Autodesk Inventor part; units mm, degrees
ref_plane "YZ Plane" through (0, 0, 0) normal (1, 0, 0) x (0, 1, 0)
ref_plane "XZ Plane" through (0, 0, 0) normal (0, 1, 0) x (-1, 0, 0)
ref_plane "XY Plane" through (0, 0, 0) normal (0, 0, 1) x (1, 0, 0)
sketch "Sketch1" plane through (0, 0, 0) normal (0, 0, 1) x (1, 0, 0)
  line L0 (-17.0246, -1.3061) -> (-17.0246, -8.9261)
  line L1 (-17.0246, -8.9261) -> (-15.272, -8.9261)
  line L2 (-15.272, -8.9261) -> (-15.272, -2.5761)
  line L3 (-15.272, -2.5761) -> (-13.8496, -2.5761)
  line L4 (-13.8496, -2.5761) -> (-13.8496, -1.9411)
  arc A0 (-13.8496, -1.9411) -> (-17.0246, -1.3061) centre (-17.0246, -9.5611) ccw
  dimension "length" = 6.35
  dimension "d1" = 0.635
  dimension "d2" = 1.27
  dimension "d3" = 1.7526
  dimension "d4" = 3.175
revolve "Revolution1" add sketch "Sketch1" angle 360 about axis through (-17.0246, -1.3061, 0) along (0, -1, 0)
ref_plane "Work Plane1" through (-17.0246, -1.3061, 0) normal (0, -1, 0) x (1, 0, 0)
sketch "Sketch2" plane through (-17.0246, -1.3061, 0) normal (0, -1, 0) x (1, 0, 0)
  line L0 (-3.0822, -0.762) -> (3.0822, -0.762)
  circle A0 centre (0, 0) radius 0.762 construction
  circle A1 centre (0, 0) radius 3.175
  line L1 (-3.0822, 0.762) -> (3.0822, 0.762)
  dimension "d8" = 1.524
extrude "Extrusion1" cut sketch "Sketch2" along normal blind 0.762 contours A1 L1 L0
thread "Thread1"
properties part number "6-32bolt" material "Brass, Soft Yellow"
For this review, take the finished solid that the model builds, in its own axes (mm). Give positions to 0.01 mm unless a question says otherwise; leave off trailing zeros. Loops run counter-clockwise (first coordinate to the right, second up) from the corner with the lowest first, then second, coordinate; pieces in that order, holes last. Notation, with made-up numbers: M 39,34 L 89,34 A13 ccw 89,46 Z; hole C 21,54.25 d9. An arc over 180 degrees is marked long. One line per item, written item: value. Start each with the question number.
Q1. Add section B-B (x = -19.25). Give the boundary of the cut face in (y, z).
Q2. For L1, parallel to Z at x = -17, y = -7; L2, parallel to Z at x = -18, y = -4; L3, parallel to X at y = -4.75, z = 1.5, list the stretches that pass through material, from the lowest coordinate up.
Q3. Add section A-A (z = 0). Give the boundary of the cut face in (x, y).
Q4. Add section D-D (x = -18.5). Give the boundary of the cut face in (y, z), and give its area (3 significant figures).
Q5. Clearance check with flat-ended pins moving along their axes: pin 1 Ø1.5 at (x, z) = (-17.5, 2.5) entering from -Y; pin 2 Ø0.8 at (x, z) = (-18.5, 0) entering from +Y; pin 3 Ø1.5 at (y, z) = (-5, -1.5) entering from +X. State where each tip first meets the part, or that it passes through.
Q6. Draft analysis for pull direction Z (two halves, no side actions). For faces 1 (the face through (-15.353, -5.707, -0.526)), 2 (the face through (-17, -2.068, 0)), 3 (the face through (-15.7, -2.576, -1.4)), state which applies: released by +Z, released by -Z, zero draft, split by the parting line, or undercut.
Q7. Add section C-C (y = -6.25). Give the boundary of the cut face in (x, z), and give its area (3 significant figures).
Reply:
1. outline: M -2.58,-2.26 L -1.94,-2.26 A7.95 ccw -1.65,-0.76 L -2.07,-0.76 L -2.07,0.76 L -1.65,0.76 A7.95 ccw -1.94,2.26 L -2.58,2.26 Z
2. L1: -1.75 to 1.75
2. L2: -1.46 to 1.46
2. L3: -17.93 to -16.12
3. outline: M -20.2,-2.58 L -18.78,-2.58 L -18.78,-8.93 L -15.27,-8.93 L -15.27,-2.58 L -13.85,-2.58 L -13.85,-2.07 L -20.2,-2.07 Z
4. outline: M -8.93,-0.95 L -2.58,-0.95 L -2.58,-2.81 L -1.94,-2.81 A8.12 ccw -1.47,-0.76 L -2.07,-0.76 L -2.07,0.76 L -1.47,0.76 A8.12 ccw -1.94,2.81 L -2.58,2.81 L -2.58,0.95 L -8.93,0.95 Z
4. area: 16.5 mm²
5. pin 1: y = -2.58
5. pin 2: y = -2.07
5. pin 3: x = -15.44
6. face 1: split by the parting line
6. face 2: undercut
6. face 3: zero draft
7. outline: C -17.02,0 d3.51
7. area: 9.65 mm²
